Autodesk Inventor part; units mm, degrees
ref_plane "YZ Plane" through (0, 0, 0) normal (1, 0, 0) x (0, 1, 0)
ref_plane "XZ Plane" through (0, 0, 0) normal (0, 1, 0) x (-1, 0, 0)
ref_plane "XY Plane" through (0, 0, 0) normal (0, 0, 1) x (1, 0, 0)
sketch "Sketch2" plane through (0, 0, 0) normal (0, 1, 0) x (-1, 0, 0)
  line L0 (0, 0) -> (150, 0)
  line L1 (150, 0) -> (150, -200)
  line L2 (150, -200) -> (0, -200)
  line L3 (0, -200) -> (0, 0)
  point P0 (75, -100)
  dimension "d4" = 150
  dimension "d5" = 200
extrude "Extrusion2" add sketch "Sketch2" along normal blind 3
sketch "Sketch3" plane through (0, 0, 0) normal (0, -1, 0) x (1, 0, 0)
  line L0 (-150, -200) -> (-150, 0)
  line L1 (-150, 0) -> (-150, -10)
  line L2 (-150, -10) -> (-147, -10)
  line L3 (-147, -10) -> (-147, -20)
  line L4 (-147, -20) -> (-150, -20)
  line L5 (-147, -30) -> (-147, -40)
  line L6 (-147, -40) -> (-150, -40)
  line L7 (-150, -30) -> (-147, -30)
  line L8 (-150, -20) -> (-150, -30)
  line L9 (-147, -50) -> (-147, -60)
  line L10 (-147, -60) -> (-150, -60)
  line L11 (-150, -50) -> (-147, -50)
  line L12 (-150, -40) -> (-150, -50)
  line L13 (-147, -70) -> (-147, -80)
  line L14 (-147, -80) -> (-150, -80)
  line L15 (-150, -70) -> (-147, -70)
  line L16 (-150, -60) -> (-150, -70)
  line L17 (-147, -90) -> (-147, -100)
  line L18 (-147, -100) -> (-150, -100)
  line L19 (-150, -90) -> (-147, -90)
  line L20 (-150, -80) -> (-150, -90)
  line L21 (-147, -110) -> (-147, -120)
  line L22 (-147, -120) -> (-150, -120)
  line L23 (-150, -110) -> (-147, -110)
  line L24 (-150, -100) -> (-150, -110)
  line L25 (-147, -130) -> (-147, -140)
  line L26 (-147, -140) -> (-150, -140)
  line L27 (-150, -130) -> (-147, -130)
  line L28 (-150, -120) -> (-150, -130)
  line L29 (-147, -150) -> (-147, -160)
  line L30 (-147, -160) -> (-150, -160)
  line L31 (-150, -150) -> (-147, -150)
  line L32 (-150, -140) -> (-150, -150)
  line L33 (-147, -170) -> (-147, -180)
  line L34 (-147, -180) -> (-150, -180)
  line L35 (-150, -170) -> (-147, -170)
  line L36 (-150, -160) -> (-150, -170)
  line L37 (-150, -180) -> (-150, -190)
  line L38 (-150, -190) -> (-147, -190)
  line L39 (0, 0) -> (0, -10)
  line L40 (0, 0) -> (0, -200)
  line L41 (-3, -10) -> (-3, -20)
  line L42 (-3, -20) -> (0, -20)
  line L43 (0, -20) -> (0, -30)
  line L44 (0, -30) -> (-3, -30)
  line L45 (-3, -30) -> (-3, -40)
  line L46 (-3, -40) -> (0, -40)
  line L47 (0, -40) -> (0, -50)
  line L48 (0, -50) -> (-3, -50)
  line L49 (-3, -50) -> (-3, -60)
  line L50 (-3, -60) -> (0, -60)
  line L51 (0, -60) -> (0, -70)
  line L52 (0, -70) -> (-3, -70)
  line L53 (-3, -70) -> (-3, -80)
  line L54 (-3, -80) -> (0, -80)
  line L55 (0, -80) -> (0, -90)
  line L56 (0, -90) -> (-3, -90)
  line L57 (-3, -90) -> (-3, -100)
  line L58 (-3, -100) -> (0, -100)
  line L59 (0, -100) -> (0, -110)
  line L60 (0, -110) -> (-3, -110)
  line L61 (-3, -110) -> (-3, -120)
  line L62 (-3, -120) -> (0, -120)
  line L63 (0, -120) -> (0, -130)
  line L64 (0, -130) -> (-3, -130)
  line L65 (-3, -130) -> (-3, -140)
  line L66 (-3, -140) -> (0, -140)
  line L67 (0, -140) -> (0, -150)
  line L68 (0, -150) -> (-3, -150)
  line L69 (-3, -150) -> (-3, -160)
  line L70 (-3, -160) -> (0, -160)
  line L71 (0, -160) -> (0, -170)
  line L72 (0, -170) -> (-3, -170)
  line L73 (-3, -170) -> (-3, -180)
  line L74 (-3, -180) -> (0, -180)
  line L75 (0, -180) -> (0, -190)
  line L76 (0, -190) -> (-3, -190)
  line L77 (-3, -190) -> (-3, -200)
  line L78 (0, -200) -> (-150, -200)
  line L79 (-147, -190) -> (-147, -200)
  line L80 (0, -10) -> (-3, -10)
  line L81 (-147, -200) -> (-140, -200)
  line L82 (-140, -197) -> (-130, -197)
  line L83 (-130, -197) -> (-130, -200)
  line L84 (-120, -200) -> (-120, -197)
  line L85 (-120, -197) -> (-110, -197)
  line L86 (-110, -197) -> (-110, -200)
  line L87 (-100, -200) -> (-100, -197)
  line L88 (-100, -197) -> (-90, -197)
  line L89 (-90, -197) -> (-90, -200)
  line L90 (-80, -200) -> (-80, -197)
  line L91 (-80, -197) -> (-70, -197)
  line L92 (-70, -197) -> (-70, -200)
  line L93 (-60, -200) -> (-60, -197)
  line L94 (-60, -197) -> (-50, -197)
  line L95 (-50, -197) -> (-50, -200)
  line L96 (-40, -200) -> (-40, -197)
  line L97 (-40, -197) -> (-30, -197)
  line L98 (-30, -197) -> (-30, -200)
  line L99 (-20, -200) -> (-20, -197)
  line L100 (-20, -197) -> (-10, -197)
  line L101 (-10, -197) -> (-10, -200)
  line L102 (-140, -197) -> (-140, -200)
  line L103 (-150, 0) -> (0, 0)
  point P0 (-10, 0)
  point P1 (-20, 0)
  dimension "d23" = 20
extrude "Extrusion3" cut sketch "Sketch3" against normal blind 3 contours L0 L34 L33 L35 L30 L29 L31 L26 L25 L27 L22 L21 L23 L18 L17 L19 L14 L13 L15 L10 L9 L11 L6 L5 L7 L4 L3 L2 L103 L39 L80 L41 L42 L40 L44 L45 L46 L48 L49 L50 L52 L53 L54 L56 L57 L58 L60 L61 L62 L64 L65 L66 L68 L69 L70 L72 L73 L74 L76 L77 L78 L101 L100 L99 L98 L97 L96 L95 L94 L93 L92 L91 L90 L89 L88 L87 L86 L85 L84 L83 L82 L102 L79 L38 keep common part
sketch "Sketch5" plane through (0, 3, 0) normal (0, 1, 0) x (1, 0, 0)
  line L0 (-150, 190) -> (-150, 0)
  circle A0 centre (-24.8562, 25.4431) radius 2.5
  circle A1 centre (-124.8562, 25.4431) radius 2.5
  circle A2 centre (-24.8562, 175.4431) radius 2.5
  circle A3 centre (-124.8562, 175.4431) radius 2.5
  point P0 (0, 0)
  point P1 (-150, 10)
  point P2 (0, 0)
  point P3 (-75, 100)
  dimension "d38" = 5
  dimension "d39" = 100
  dimension "d40" = 150
extrude "Extrusion4" cut sketch "Sketch5" against normal blind 2
properties part number "TableBottom" material "Wood (Cherry)"
Read the model definition and answer for the solid it produces. Units are mm, in the model's axes. A direction names the side the tool comes from. Round coordinates to 2 decimals unless told otherwise and drop trailing zeros. Write each loop counter-clockwise with the first axis right and the second up, starting at its lowest first coordinate (ties: lowest second). Pieces come first, ordered by that corner, then holes.
Q1. The mould has two halves that part along Z. Classify faces 1 (the face through (-74, 3, -99)), 2 (the face through (-125, 1, -25)): released by +Z, released by -Z, zero draft, split by the parting line, or undercut.
Values:
face 1: zero draft
face 2: undercut
Q2. Flat-ended cylindrical pins translate along their axes: P1, Ø1.5, axis at y = 2, z = -198.5, coming from the +X side; P2, Ø4, axis at x = -125, z = -175, coming from the +Y side; P3, Ø0.9, axis at y = 2, z = -97, coming from the -X side. Find the tip coordinate at first contact, or state that the pin passes through.
Values:
P1: stops at x = -3
P2: stops at y = 1
P3: stops at x = -147
Q3. Find section A-A on z = -74. Determine the outline of the cut face in (x, y).
Values:
outline: (-147, 0) - (-3, 0) - (-3, 3) - (-147, 3) - close
Q4. Straight lines are drawn through the part: line 1 (X direction, y = 2.8, z = -177); line 2 (Z direction, x = -99.5, y = 2.2); line 3 (X direction, y = 1.65, z = -34). For each, find the intervals that lie inside material, in ascending order.
Values:
line 1: x = -147 to -126.81, -122.9 to -26.81, -22.9 to -3
line 2: z = -197 to 0
line 3: x = -147 to -3
Q5. A tool of negligible diameter and unlimited length cuts with its end or side. For faces 3 (the face through (-74, 0, -99)), 4 (the face through (-122.547, 2.014, -174.486)), from which of +Z, -Z, +X, -X, +Y, -Y can it reach the whole face along a straight path? Write none if from no direction.
Values:
face 3: +Z, -Z, +X, -X, -Y
face 4: +Y
Q6. Find section B-B on x = -16.5. Determine the outline of the cut face in (y, z).
Values:
outline: (0, -197) - (3, -197) - (3, 0) - (0, 0) - close
Q7. Find section C-C on y = 2.45. State how many separate pieces and enclosed holes the cut face has, and give its area (3 significant figures).
Values:
separate pieces: 1
enclosed holes: 4
area: 29,100 mm2
